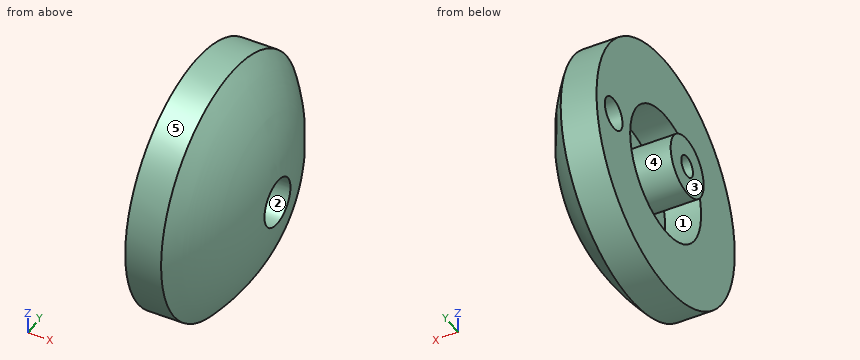
Autodesk Inventor part; units mm, degrees
ref_plane "Work Plane3" through (3.9124, 0, 0) normal (1, 0, 0) x (0, 1, 0)
ref_plane "Work Plane4" through (-2.921, 0, 0) normal (-1, 0, 0) x (0, 0, 1)
ref_plane "XZ Plane" through (0, 0, 0) normal (0, 1, 0) x (-1, 0, 0)
sketch "Sketch1" plane through (0, 0, 0) normal (0, 0, 1) x (1, 0, 0)
  line L0 (0, 0) -> (-8.052, 0) construction
  line L1 (-6.096, 2.032) -> (5.08, 2.032)
  line L2 (-6.096, 2.032) -> (-6.096, 3.2258)
  line L3 (-6.096, 3.2258) -> (0, 3.2258)
  line L4 (0, 3.2258) -> (0, 6.9342)
  line L5 (0, 6.9342) -> (-3.81, 6.9342)
  line L6 (-3.81, 6.9342) -> (-3.81, 13.5128)
  line L7 (-3.81, 13.5128) -> (0, 13.5128)
  arc A0 (5.08, 2.032) -> (0, 13.5128) centre (-15.0256, 0) ccw
  dimension "d0" = 2.032
  dimension "d1" = 13.5128
  dimension "d2" = 6.096
  dimension "d3" = 3.2258
  dimension "d4" = 3.81
  dimension "d5" = 6.9342
  dimension "d7" = 5.08
revolve "Revolution1" add sketch "Sketch1" angle 360 about axis through (0, 0, 0) along (-1, 0, 0)
ref_plane "Work Plane3" through (3.9124, 0, 0) normal (1, 0, 0) x (0, 1, 0)
ref_plane "Work Plane2" through (5.1824, 0, 0) normal (1, 0, 0) x (0, 1, 0)
sketch "Sketch4" plane through (-3.81, 0, 0) normal (-1, 0, 0) x (0, 0, 1)
  circle A0 centre (0, 10.16) radius 1.7272
extrude "Extrusion3" cut sketch "Sketch4" against normal through all
sketch "Sketch5" plane through (-6.096, 0, 0) normal (-1, 0, 0) x (0, 0, 1)
  circle A0 centre (0, 0) radius 2.032
  circle A1 centre (0, 0) radius 3.2258
  circle A2 centre (0, 0) radius 1.143
  dimension "d18" = 2.286
extrude "Extrusion4" add sketch "Sketch5" against normal up to surface contours A0
ref_plane "Work Plane4" through (-2.921, 0, 0) normal (-1, 0, 0) x (0, 0, 1)
sketch "Sketch6" plane through (-2.921, 0, 0) normal (-1, 0, 0) x (0, 0, 1)
  circle A0 centre (0, 0) radius 2.54
  dimension "d22" = 5.08
extrude "Extrusion5" cut sketch "Sketch6" against normal through all
chamfer "Chamfer1" distance 1.27 angle 45 1 edges at (-2.921, 0, -1.143)
properties part number "Flexiwheel Hub - Out Side"
Can you work these out from the model? Positions are in its coordinate system, mm. Face numbers are marked on the shaded views. A direction names the side the tool comes from. Give positions to 0.01 mm unless a question says otherwise; leave off trailing zeros. Loops run counter-clockwise (first coordinate to the right, second up) from the corner with the lowest first, then second, coordinate; pieces in that order, holes last. Notation, with made-up numbers: (-21, 14) - (14, 14) arc R6 cw to (14, 20) - close; hole circle Ø1 at (6.5, 29.25). An arc over 180 degrees is marked (long way). Return JSON: item names as keys, results as strings.
1. I want a section at A-A on x = -2. Please give me the cut outline in (y, z), and give its area (3 significant figures).
Output values:
{"outline": "circle Ø27.03 at (0, 0); circle Ø6.45 at (0, 0); hole circle Ø13.87 at (0, 0); hole circle Ø5.08 at (0, 0); hole circle Ø3.45 at (10.16, 0)", "area": "426 mm²"}
2. We'd pull the mould along Z, two halves only. Please class the marked faces 3, 4 and 5: +Z half, -Z half, draft (parallel to the pull), parting line (faces both ways), or undercut.
Output values:
{"face 3": "draft", "face 4": "undercut", "face 5": "parting line"}
3. I want a section at B-B on z = 0. Give the number of separate pieces and of enclosed holes in the cut face, and give its area (3 significant figures).
Output values:
{"separate pieces": "3", "enclosed holes": "0", "area": "114 mm²"}
4. For the marked faces 1 and 2, which set-ups out of +Z, -Z, +X, -X, +Y, -Y let a thin tool reach every point of the face, with its end or its side?
Output values:
{"face 1": "-X", "face 2": "+X"}
5. If I drill on line 1 (Z direction, x = -2.6, y = 0); line 2 (Y direction, x = -1.25, z = 0); line 3 (Y direction, x = -0.75, z = -1.25), over which ranges is the centre line in solid material (lowest first)?
Output values:
{"line 1": "z = -13.51 to -6.93, -3.23 to -2.54, 2.54 to 3.23, 6.93 to 13.51", "line 2": "y = -13.51 to -6.93, -3.23 to -2.54, 2.54 to 3.23, 6.93 to 8.43, 11.89 to 13.51", "line 3": "y = -13.45 to -6.82, -2.97 to -2.21, 2.21 to 2.97, 6.82 to 8.97, 11.35 to 13.45"}
6. I'm going to push flat-ended pins straight in: pin 1 Ø4 at (y, z) = (0, 0) entering from -X; pin 2 Ø1.5 at (y, z) = (0, -0.5) entering from +X; pin 3 Ø5 at (x, y) = (0.5, 9) entering from +Z; pin 4 Ø8 at (y, z) = (-8.5, -7) entering from -X. Where does each tip first touch, or does it pass through?
Output values:
{"pin 1": "stops at x = -6.1", "pin 2": "stops at x = -4.08", "pin 3": "stops at z = 11.82", "pin 4": "stops at x = -3.81"}
